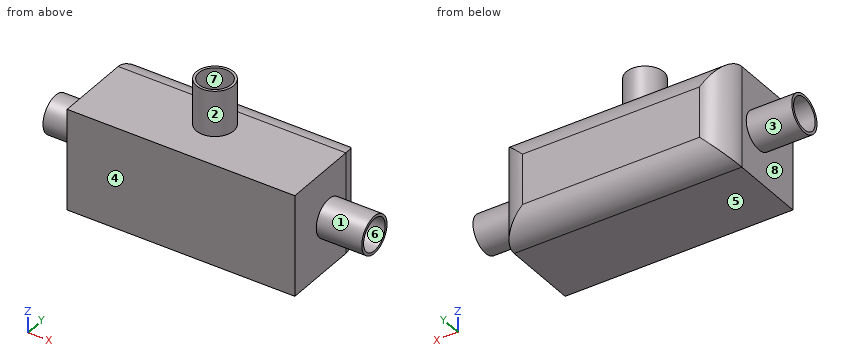
```python
from build123d import *

# Parameters (mm, degrees)
CROQUIS1_W              = 90
CROQUIS1_H              = 40
SALIENTE_EXTRUIR1_DEPTH = 40
CROQUIS2_R              = 7.421380831
CROQUIS2_R_2            = 6.35
SALIENTE_EXTRUIR2_DEPTH = 18
SALIENTE_EXTRUIR3_START = 18
CROQUIS3_R              = 7.421380831
CROQUIS3_R_2            = 6.35
SALIENTE_EXTRUIR3_DEPTH = 18
CROQUIS4_R              = 7.356347307
CROQUIS4_R_2            = 6.35
SALIENTE_EXTRUIR4_DEPTH = 18
REDONDEO1_R             = 10


with BuildPart() as part:
    # Croquis1 → Saliente-Extruir1 (new body)
    with BuildSketch(Plane(origin=(0, 0, 0), x_dir=(1, 0, 0), z_dir=(0, 1, 0))):
        Rectangle(CROQUIS1_W, CROQUIS1_H)
    extrude(amount=SALIENTE_EXTRUIR1_DEPTH)

    # Croquis2 → Saliente-Extruir2 (add)
    with BuildSketch(Plane(origin=(45, 0, 0), x_dir=(0, 0, -1), z_dir=(1, 0, 0))):
        with Locations(Location((0, 20, 0), (0, 0, 180))):
            Circle(CROQUIS2_R)
        with Locations((0, 20)):
            Circle(CROQUIS2_R_2, mode=Mode.SUBTRACT)
    extrude(amount=SALIENTE_EXTRUIR2_DEPTH)

    # Croquis3 → Saliente-Extruir3 (add)
    with BuildSketch(Plane.ZY.offset(45).offset(SALIENTE_EXTRUIR3_START)):
        with Locations((0, 20)):
            Circle(CROQUIS3_R)
        with Locations(Location((0, 20, 0), (0, 0, 180))):
            Circle(CROQUIS3_R_2, mode=Mode.SUBTRACT)
    extrude(amount=-SALIENTE_EXTRUIR3_DEPTH)

    # Croquis4 → Saliente-Extruir4 (add)
    with BuildSketch(Plane.XY.offset(20)):
        with Locations(Location((0, 20, 0), (0, 0, 180))):
            Circle(CROQUIS4_R)
        with Locations((0, 20)):
            Circle(CROQUIS4_R_2, mode=Mode.SUBTRACT)
    extrude(amount=SALIENTE_EXTRUIR4_DEPTH)

    # Redondeo1
    redondeo1_edges = [part.edges().sort_by_distance(p)[0] for p in [
        (-45, 40, 0),
        (0, 40, 20),
        (45, 40, 0),
        (0, 40, -20),
    ]]
    fillet(redondeo1_edges, radius=REDONDEO1_R)


solid = part.part
```
Can you work these out from the model? Positions are in its coordinate system, mm. Face numbers are marked on the shaded views. A direction names the side the tool comes from. Give positions to 0.01 mm unless a question says otherwise; leave off trailing zeros. Write each loop counter-clockwise with the first axis right and the second up, starting at its lowest first coordinate (ties: lowest second). Pieces come first, ordered by that corner, then holes. Notation, with made-up numbers: (23, 68) - (81, 68) arc R14 cw to (81, 80) - close; hole circle Ø1 at (-5, 47.5). An arc over 180 degrees is marked (long way). Write item = value, one per line. Start each with the question number.
1. Please list where these lines run through material, in increasing order: line 1 (Y direction, x = -51.75, z = 0); line 2 (Z direction, x = 3, y = 2.5); line 3 (X direction, y = 5, z = -7.5).
2. Imagine slicing it at C-C (y = 20). Please give me the cut outline in (x, z).
3. For pin 1 (8 mm diameter, centred on y = 24.5, z = -13, fed in from +X); pin 2 (8 mm diameter, centred on x = -25, z = 23, fed in from +Y); pin 3 (2 mm diameter, centred on y = 16, z = 21.5, fed in from -X), each with a flat end and sliding along its axis, tell me the tip position at first contact or that it passes through.
4. Imagine slicing it at B-B (z = 0). Please give me the cut outline in (x, y), and give its area (3 significant figures).
5. Imagine slicing it at A-A (x = 0). Please give me the cut outline in (y, z).
6. On a 3-axis mill with a long thin cutter (end or side, diameter ignored), from which of +Z, -Z, +X, -X, +Y, -Y can I reach the whole of each face in a straight line? I mean the marked faces 1, 2, 3, 4 and 5. Say none if no direction works.
7. Imagine slicing it at D-D (z = 31). Please give me the cut outline in (x, y).
8. Thinking about a two-plate mould opening in X: for the marked faces 6, 7 and 8, which applies, released by +X, released by -X, zero draft, split by the parting line, or undercut?
Worked answers:
q1.line_1 = 12.58 to 13.65, 26.35 to 27.42
q1.line_2 = -20 to 20
q1.line_3 = -45 to 45
q2.outline = (-63, -7.42) - (-45, -7.42) - (-45, -20) - (45, -20) - (45, -7.42) - (63, -7.42) - (63, -6.35) - (45, -6.35) - (45, 6.35) - (63, 6.35) - (63, 7.42) - (45, 7.42) - (45, 20) - (7.36, 20) - (7.36, 38) - (6.35, 38) - (6.35, 20) - (-6.35, 20) - (-6.35, 38) - (-7.36, 38) - (-7.36, 20) - (-45, 20) - (-45, 7.42) - (-63, 7.42) - (-63, 6.35) - (-45, 6.35) - (-45, -6.35) - (-63, -6.35) - close
q3.pin_1 = 45
q3.pin_2 = 34.36
q3.pin_3 = -6.72
q4.outline = (-63, 12.58) - (-45, 12.58) - (-45, 0) - (45, 0) - (45, 12.58) - (63, 12.58) - (63, 13.65) - (45, 13.65) - (45, 26.35) - (63, 26.35) - (63, 27.42) - (45, 27.42) - (45, 30) arc R10 ccw to (35, 40) - (-35, 40) arc R10 ccw to (-45, 30) - (-45, 27.42) - (-63, 27.42) - (-63, 26.35) - (-45, 26.35) - (-45, 13.65) - (-63, 13.65) - close
q4.area = 3,630 mm2
q5.outline = (0, -20) - (30, -20) arc R10 ccw to (40, -10) - (40, 10) arc R10 ccw to (30, 20) - (27.36, 20) - (27.36, 38) - (26.35, 38) - (26.35, 20) - (13.65, 20) - (13.65, 38) - (12.64, 38) - (12.64, 20) - (0, 20) - close
q6.face_1 = +X
q6.face_2 = +Z
q6.face_3 = -X
q6.face_4 = +Z, -Z, +X, -X, -Y
q6.face_5 = -Z, +X, -X, +Y, -Y
q7.outline = circle Ø14.71 at (0, 20); hole circle Ø12.7 at (0, 20)
q8.face_6 = zero draft
q8.face_7 = undercut
q8.face_8 = released by -X
